Can you work these out from the model? Positions are in its coordinate system, mm. A direction names the side the tool comes from. Coordinates: 2 decimals unless noted, no trailing zeros. Loops run counter-clockwise (first coordinate to the right, second up) from the corner with the lowest first, then second, coordinate; pieces in that order, holes last. Notation, with made-up numbers: M 78,63.25 L 95,63.25 A31 ccw 95,95.25 Z; hole C 18,-9.5 d6. An arc over 180 degrees is marked long. Answer as a JSON object with one key per item and string values. Group by question number.
Item 1: We'd pull the mould along Z, two halves only. Please class faces 1 (the flat face through (25, 0, 1)), 2 (the flat face through (25, -852, 0)), 3 (the flat face through (25, -852, 1.587)): +Z half, -Z half, draft (parallel to the pull), parting line (faces both ways), or undercut.
Item 2: If I drill on line 1 (Z direction, x = 40, y = -524), over which ranges is the centre line in solid material (lowest first)?
Item 3: Suppose I cut it at B-B (z = 33.5). Write out the boundary of the cut face in (x, y).
Item 4: Suppose I cut it at A-A (x = 20). Write out the boundary of the cut face in (y, z), then the cut area to 3 significant figures.
Item 5: Which directions (+Z, -Z, +X, -X, +Y, -Y) give clear straight access to the entire face, cutting with the end or side of a thin tool? Please do faces 4 (the flat face through (25, -852, 50.8)), 5 (the flat face through (1.587, -852, 25)).
```python
from build123d import *

# Parameters (mm, degrees)
F0_W     = 50.8
F0_H     = 50.8
F0_W_2   = 47.625
F0_H_2   = 47.625
F1_DEPTH = 1727.2
F2_R     = 3.175
F3_R     = 1.5875


with BuildPart() as f1:
    # F0 (on Front) → F1 (new body)
    with BuildSketch(Plane.XZ):
        with Locations((25.4, 25.4)):
            Rectangle(F0_W, F0_H)
        with Locations((25.4, 25.4)):
            Rectangle(F0_W_2, F0_H_2, mode=Mode.SUBTRACT)
    extrude(amount=F1_DEPTH)

    # F2
    f2_edges = [f1.edges().sort_by_distance(p)[0] for p in [
        (0, -863.6, 50.8),
        (50.8, -863.6, 50.8),
        (50.8, -863.6, 0),
        (0, -863.6, 0),
    ]]
    fillet(f2_edges, radius=F2_R)

    # F3
    f3_edges = [f1.edges().sort_by_distance(p)[0] for p in [
        (1.5875, -863.6, 49.2125),
        (49.2125, -863.6, 49.2125),
        (1.5875, -863.6, 1.5875),
        (49.2125, -863.6, 1.5875),
    ]]
    fillet(f3_edges, radius=F3_R)


solid = f1.part
```
From the geometry:
{
 "1": {"face 1": "draft", "face 2": "-Z half", "face 3": "undercut"},
 "2": {"line 1": "0 to 1.59, 49.21 to 50.8"},
 "3": {"outline": "M 0,-1727.2 L 1.59,-1727.2 L 1.59,0 L 0,0 Z; M 49.21,-1727.2 L 50.8,-1727.2 L 50.8,0 L 49.21,0 Z"},
 "4": {"outline": "M -1727.2,0 L 0,0 L 0,1.59 L -1727.2,1.59 Z; M -1727.2,49.21 L 0,49.21 L 0,50.8 L -1727.2,50.8 Z", "area": "5,480 mm2"},
 "5": {"face 4": "+Z, +X, -X, +Y, -Y", "face 5": "+Y, -Y"}
}
